Verification items for the finished model (mm, model axes). Coordinates: 2 decimals unless noted, no trailing zeros. Order: outer loops, then holes, each group sorted by start corner. A loop starts at its lowest first (then second) coordinate and runs counter-clockwise, first axis right, second up. Notation, with made-up numbers: (63, 28.25) -> (76, 28.25) arc R33 cw to (76, 67.25) -> close; hole circle Ø2 at (72, -13.75). An arc over 180 degrees is marked (long way). Use CSV: the item, a comma, the result in double quotes. Start each with the question number.
1) Scan lines: line 1 along Z through (x, y) = (6.5, -16.5); line 2 along Y through (x, z) = (18, -4); line 3 along Z through (x, y) = (-8.5, -39). Record each from-to range of solid material in increasing order.
2) Sectioned sample at C-C on x = 16. Record the boundary of the cut face in (y, z).
3) Sectioned sample at D-D on y = 70. Record the boundary of the cut face in (x, z), then the cut area to 3 significant figures.
4) Sectioned sample at A-A on y = -70. Record the boundary of the cut face in (x, z), then the cut area to 3 significant figures.
5) Sectioned sample at B-B on z = -47. Record the boundary of the cut face in (x, y), then the cut area to 3 significant figures.
6) Go/stop test with flat-tipped pins: pin 1 (5 mm diameter, centred on x = 6.5, z = -42, fed in from +Y); pin 2 (4 mm diameter, centred on x = 8, y = 78, fed in from +Z); pin 3 (2.5 mm diameter, centred on x = -1, z = 63.5, fed in from +Y). Record where each tip stops, or that it passes through.
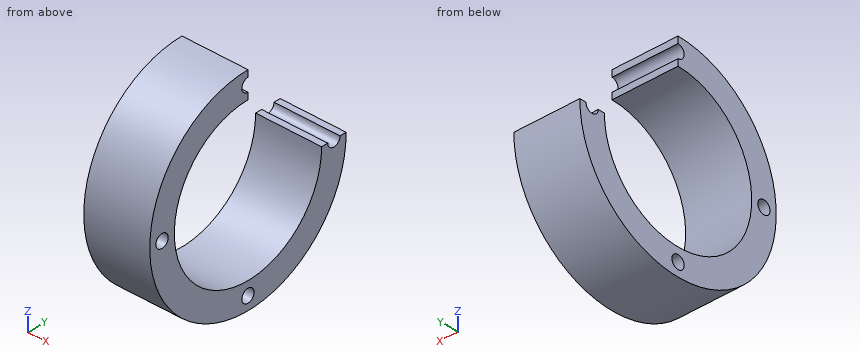
from build123d import *

# Parameters (mm, degrees)
SKETCH1_R           = 80
SKETCH1_R_2         = 60
BOSS_EXTRUDE1_DEPTH = 25
SKETCH2_R           = 5
CUT_EXTRUDE1_DEPTH  = 124.693168769
CIRPATTERN1_COUNT   = 4
CUT_EXTRUDE2_DEPTH  = 124.693168769


with BuildPart() as part:
    # Sketch1 → Boss-Extrude1 (new, symmetric)
    with BuildSketch(Plane.YZ):
        with Locations(Location((0, 0, 0), (0, 0, 270))):
            Circle(SKETCH1_R)
        with Locations(Location((0, 0, 0), (0, 0, 270))):
            Circle(SKETCH1_R_2, mode=Mode.SUBTRACT)
    extrude(amount=BOSS_EXTRUDE1_DEPTH, both=True)

    # Sketch2 → Cut-Extrude1 (cut, through all)
    with BuildSketch(Plane.YZ.offset(25)):
        with Locations(Location((-70, 0, 0), (0, 0, 270))):
            Circle(SKETCH2_R)
    cut_extrude1 = extrude(amount=-CUT_EXTRUDE1_DEPTH, mode=Mode.SUBTRACT)

    # CirPattern1: Cut-Extrude1 ×4 about axis
    cirpattern1_axis = Axis((0, 0, 0), (1, 0, 0))
    for i in range(1, CIRPATTERN1_COUNT):
        add(cut_extrude1.rotate(cirpattern1_axis, i * 360 / CIRPATTERN1_COUNT), mode=Mode.SUBTRACT)

    # Sketch3 → Cut-Extrude2 (cut, through all)
    with BuildSketch(Plane.YZ.offset(25)):
        Polygon((0, 93.474358871), (0, 0), (100.664694168, 0), (100.664694168, 96.534076019), align=None)
    extrude(amount=-CUT_EXTRUDE2_DEPTH, mode=Mode.SUBTRACT)


solid = part.part
Answers follow:
1,line 1,"z = -78.28 to -57.69, 57.69 to 78.28"
1,line 2,"y = -79.9 to -73, -67 to -59.87, 59.87 to 67, 73 to 79.9"
1,line 3,"z = -69.85 to -45.6, 45.6 to 69.85"
2,outline,"(0, 60) -> (0, 65) arc R5 cw to (0, 75) -> (0, 80) arc R80 ccw (long way) to (80, 0) -> (75, 0) arc R5 cw to (65, 0) -> (60, 0) arc R60 cw (long way) to start; hole circle Ø10 at (-70, 0); hole circle Ø10 at (0, -70)"
3,outline,"(-25, -38.73) -> (25, -38.73) -> (25, -5) -> (-25, -5) -> close"
3,area,"1,690 mm²"
4,outline,"(-25, -38.73) -> (25, -38.73) -> (25, -5) -> (-25, -5) -> close; (-25, 5) -> (25, 5) -> (25, 38.73) -> (-25, 38.73) -> close"
4,area,"3,370 mm²"
5,outline,"(-25, -64.74) -> (25, -64.74) -> (25, -37.3) -> (-25, -37.3) -> close; (-25, 37.3) -> (25, 37.3) -> (25, 64.74) -> (-25, 64.74) -> close"
5,area,"2,740 mm²"
6,pin 1,"stops at y = 69.57"
6,pin 2,"stops at z = 0"
6,pin 3,"stops at y = 0"
